from build123d import *

# Parameters (mm, degrees)
SKETCH_1_W          = 120
SKETCH_1_H          = 65
EXTRUDE_1_DEPTH     = 3
SKETCH_2_R          = 1.6
CUT_EXTRUDE_1_DEPTH = 137.506410106
FILLET_1_R          = 5
SKETCH_3_R          = 23.5
CUT_EXTRUDE_2_DEPTH = 10
SKETCH_4_R          = 2.1
CUT_EXTRUDE_3_DEPTH = 5


with BuildPart() as part:
    # 草图1 → 凸台-拉伸1 (new body)
    with BuildSketch(Plane.XY):
        with Locations((60, -32.5)):
            Rectangle(SKETCH_1_W, SKETCH_1_H)
    extrude(amount=EXTRUDE_1_DEPTH)

    # 草图2 → 切除-拉伸1 (cut, through all)
    with BuildSketch(Plane.XY.offset(3)):
        with Locations((10, -5)):
            Circle(SKETCH_2_R)
        with Locations((10, -32.5)):
            Circle(SKETCH_2_R)
        with Locations((10, -60)):
            Circle(SKETCH_2_R)
        with Locations(Location((110, -60, 0), (0, 0, 180))):
            Circle(SKETCH_2_R)
        with Locations(Location((110, -32.5, 0), (0, 0, 180))):
            Circle(SKETCH_2_R)
        with Locations(Location((110, -5, 0), (0, 0, 180))):
            Circle(SKETCH_2_R)
    extrude(amount=-CUT_EXTRUDE_1_DEPTH, mode=Mode.SUBTRACT)

    # 圆角1
    fillet_1_edges = [part.edges().sort_by_distance(p)[0] for p in [
        (0, 0, 1.5),
        (120, 0, 1.5),
        (120, -65, 1.5),
        (0, -65, 1.5),
    ]]
    fillet(fillet_1_edges, radius=FILLET_1_R)

    # 草图3 → 切除-拉伸2 (cut)
    with BuildSketch(Plane.XY.offset(3)):
        with Locations((60, -32.5)):
            Circle(SKETCH_3_R)
    extrude(amount=-CUT_EXTRUDE_2_DEPTH, mode=Mode.SUBTRACT)

    # 草图4 → 切除-拉伸3 (cut, symmetric)
    with BuildSketch(Plane.XY.offset(3)):
        with Locations((84.04163056, -8.45836944)):
            Circle(SKETCH_4_R)
        with Locations((84.04163056, -56.54163056)):
            Circle(SKETCH_4_R)
        with Locations((35.95836944, -56.54163056)):
            Circle(SKETCH_4_R)
        with Locations((35.95836944, -8.45836944)):
            Circle(SKETCH_4_R)
    extrude(amount=CUT_EXTRUDE_3_DEPTH, both=True, mode=Mode.SUBTRACT)


solid = part.part
CAD build for the part. Positions are in the model's coordinates, mm. Round coordinates to 2 decimals unless told otherwise and drop trailing zeros. Loops run counter-clockwise (first coordinate to the right, second up) from the corner with the lowest first, then second, coordinate; pieces in that order, holes last. Notation, with made-up numbers: (51.5, -36) - (95.5, -36) arc R25 ccw to (95.5, 3) - close; hole circle Ø9 at (66, 74). An arc over 180 degrees is marked (long way). Put each result on its own line as item: value.
1. Two-plate mould, pull along Y, no slides. Class faces 1 (the flat face through (0, -33, 1)), 2 (the cylindrical face through (8.4, -4.93, 1.52)), 3 (the cylindrical face through (8.73, -33.47, 1.52)), 4 (the flat face through (59, 0, 1)): released by +Y, released by -Y, zero draft, split by the parting line, or undercut.
Geometry check:
face 1: zero draft
face 2: undercut
face 3: undercut
face 4: released by +Y
2. Wall check: line 1 (Y direction, x = 110, z = 2.35); line 2 (Y direction, x = 61, z = 2.7); line 3 (Y direction, x = 35, z = 2.45). Give the ranges that are in metal, low to high.
Geometry check:
line 1: -65 to -61.6, -58.4 to -34.1, -30.9 to -6.6, -3.4 to 0
line 2: -65 to -55.98, -9.02 to 0
line 3: -65 to -58.41, -54.67 to -10.33, -6.59 to 0
3. Slice it at A-A on y = -32.5. List the corners of the cut face in (x, z), and give its area (3 significant figures).
Geometry check:
outline: (0, 0) - (8.4, 0) - (8.4, 3) - (0, 3) - close; (11.6, 0) - (36.5, 0) - (36.5, 3) - (11.6, 3) - close; (83.5, 0) - (108.4, 0) - (108.4, 3) - (83.5, 3) - close; (111.6, 0) - (120, 0) - (120, 3) - (111.6, 3) - close
area: 200 mm²
4. Slice it at B-B on x = 10. List the corners of the cut face in (y, z), and give its area (3 significant figures).
Geometry check:
outline: (-65, 0) - (-61.6, 0) - (-61.6, 3) - (-65, 3) - close; (-58.4, 0) - (-34.1, 0) - (-34.1, 3) - (-58.4, 3) - close; (-30.9, 0) - (-6.6, 0) - (-6.6, 3) - (-30.9, 3) - close; (-3.4, 0) - (0, 0) - (0, 3) - (-3.4, 3) - close
area: 166 mm²
5. Slice it at D-D on x = 60. List the corners of the cut face in (y, z).
Geometry check:
outline: (-65, 0) - (-56, 0) - (-56, 3) - (-65, 3) - close; (-9, 0) - (0, 0) - (0, 3) - (-9, 3) - close
6. Slice it at C-C on y = -15. List the corners of the cut face in (x, z), and give its area (3 significant figures).
Geometry check:
outline: (0, 0) - (44.32, 0) - (44.32, 3) - (0, 3) - close; (75.68, 0) - (120, 0) - (120, 3) - (75.68, 3) - close
area: 266 mm²
